Read the model definition and answer for the solid it produces. Units are mm, in the model's axes. A direction names the side the tool comes from. Coordinates: 2 decimals unless noted, no trailing zeros. Order: outer loops, then holes, each group sorted by start corner. A loop starts at its lowest first (then second) coordinate and runs counter-clockwise, first axis right, second up. Notation, with made-up numbers: (-12.5, 42) -> (2.5, 42) arc R33 ccw to (2.5, 70) -> close; hole circle Ø1 at (63.25, 36). An arc over 180 degrees is marked (long way). Use CSV: the item, a comma, the result in double quotes.
```python
from build123d import *

# Parameters (mm, degrees)
F2_DEPTH = 12.7
F0_R     = 2.54
F3_DEPTH = 25.4
F4_R     = 2.54
F5_SIZE  = 1.27


with BuildPart() as f2:
    # F1 (on Right) → F2 (new body)
    with BuildSketch(Plane.YZ):
        with BuildLine():
            Line((4.7625, 0), (4.7625, -4.7625))
            ThreePointArc((4.7625, -4.7625), (0, -9.525), (-4.7625, -4.7625))
            Line((-4.7625, -4.7625), (-4.7625, 0))
            Line((-4.7625, 0), (-19.05, 0))
            Line((-19.05, 0), (-19.05, -12.7))
            Line((-19.05, -12.7), (-7.77713, -12.7))
            ThreePointArc((-7.77713, -12.7), (0, -15.875), (7.77713, -12.7))
            Line((7.77713, -12.7), (19.05, -12.7))
            Line((19.05, -12.7), (19.05, 0))
            Line((19.05, 0), (4.7625, 0))
        make_face()
    extrude(amount=F2_DEPTH)

    # F0 (on Top) → F3 (cut)
    with BuildSketch(Plane.XY):
        with Locations((6.35, 12.7)):
            Circle(F0_R)
        with Locations((6.35, -12.7)):
            Circle(F0_R)
        with BuildLine():
            ThreePointArc((0, -9.984122), (4.850968, 0), (0, 9.984122))
            Line((0, 9.984122), (0, -9.984122))
        make_face()
    extrude(amount=-F3_DEPTH, mode=Mode.SUBTRACT)

    # F4
    f4_edges = [f2.edges().sort_by_distance(p)[0] for p in [
        (6.35, 19.05, -12.7),
        (6.35, -19.05, -12.7),
        (7.4456, 7.77713, -12.7),
        (7.4456, -7.77713, -12.7),
    ]]
    fillet(f4_edges, radius=F4_R)

    # F5
    f5_edges = [f2.edges().sort_by_distance(p)[0] for p in [
        (3.81, 12.7, -12.7),
        (3.81, -12.7, -12.7),
    ]]
    chamfer(f5_edges, length=F5_SIZE)


solid = f2.part
```
Item 1: Straight lines are drawn through the part: line 1 along Y through (x, z) = (6.35, -4); line 2 along Y through (x, z) = (6.25, -10.25); line 3 along Y through (x, z) = (5.25, -2.5). For each, find the intervals that lie inside material, in ascending order.
Return value:
line 1,"y = -19.05 to -15.24, -10.16 to -4.76, 4.76 to 10.16, 15.24 to 19.05"
line 2,"y = -19.05 to -15.24, -10.16 to 10.16, 15.24 to 19.05"
line 3,"y = -19.05 to -14.99, -10.41 to -4.76, 4.76 to 10.41, 14.99 to 19.05"
Item 2: The mould has two halves that part along X. Classify faces 4 (the cylindrical face through (6.02, 15.22, -5.63)), 5 (the flat face through (0, 14, -6)), 6 (the cylindrical face through (7.106, 7.898, -12.848)), 7 (the flat face through (12.7, 0, -10)): +X half, -X half, draft (parallel to the pull), parting line (faces both ways), or undercut.
Return value:
face 4,"undercut"
face 5,"-X half"
face 6,"draft"
face 7,"+X half"
Item 3: Find section D-D, the plane y = 0. Give the vertices of the cut face in (x, z) (3 decimals), then the cut area to 3 significant figures.
Return value:
outline,"(4.851, -15.875) -> (12.7, -15.875) -> (12.7, -9.525) -> (4.851, -9.525) -> close"
area,"49.8 mm^2"
Item 4: Find section B-B, the plane y = 12.7. Give the vertices of the cut face in (x, z), then the cut area to 3 significant figures.
Return value:
outline,"(0, -12.7) -> (2.54, -12.7) -> (3.81, -11.43) -> (3.81, 0) -> (0, 0) -> close; (8.89, -11.43) -> (10.16, -12.7) -> (12.7, -12.7) -> (12.7, 0) -> (8.89, 0) -> close"
area,"95.2 mm^2"
Item 5: Find section C-C, the plane z = -5.25. Give the vertices of the cut face in (x, y), then the cut area to 3 significant figures.
Return value:
outline,"(0, -19.05) -> (12.7, -19.05) -> (12.7, -4.74) -> (3.93, -4.74) arc R12.7 cw to (0, -9.98) -> close; (0, 9.98) arc R12.7 cw to (3.93, 4.74) -> (12.7, 4.74) -> (12.7, 19.05) -> (0, 19.05) -> close; hole circle Ø5.08 at (6.35, -12.7); hole circle Ø5.08 at (6.35, 12.7)"
area,"299 mm^2"
Item 6: Find section A-A, the plane z = -2.5. Give the vertices of the cut face in (x, y), then the cut area to 3 significant figures.
Return value:
outline,"(0, -19.05) -> (12.7, -19.05) -> (12.7, -4.76) -> (3.92, -4.76) arc R12.7 cw to (0, -9.98) -> close; (0, 9.98) arc R12.7 cw to (3.92, 4.76) -> (12.7, 4.76) -> (12.7, 19.05) -> (0, 19.05) -> close; hole circle Ø5.08 at (6.35, -12.7); hole circle Ø5.08 at (6.35, 12.7)"
area,"298 mm^2"
Item 7: Each of these flat-tipped pins is pushed along its axis until it touches: P1, Ø4.5, axis at x = 6.35, y = 12.7, coming from the -Z side; P2, Ø6, axis at x = 4, y = 13, coming from the -Z side; P3, Ø4, axis at x = 7, y = 13, coming from the -Z side. Where does it stop, or does it pass through?
Return value:
P1,"passes through"
P2,"stops at z = -12.7"
P3,"stops at z = -11.61"
Item 8: A tool of negligible diameter and unlimited length cuts with its end or side. For faces 1 (the cylindrical face through (6.439, 18.286, -11.976)), 2 (the flat face through (8, -4.762, -2)), 3 (the flat face through (3, -15, -12.7)), from which of +Z, -Z, +X, -X, +Y, -Y can it reach the whole face along a straight path? Write none if from no direction.
Return value:
face 1,"-Z, +X, -X, +Y"
face 2,"+Z, +X, -X"
face 3,"-Z, +X, -X, -Y"
